Part model, mm, in its own coordinate system. A direction names the side the tool comes from. Give positions to 0.01 mm unless a question says otherwise; leave off trailing zeros. Order: outer loops, then holes, each group sorted by start corner. A loop starts at its lowest first (then second) coordinate and runs counter-clockwise, first axis right, second up. Notation, with made-up numbers: M 10,23.5 L 45,23.5 A18 ccw 45,46.5 Z; hole C -15,48 d3. An arc over 180 degrees is marked long. Answer as a JSON object with one key per item and string values.
from build123d import *

# Parameters (mm, degrees)
HEX_START   = -2.8194
HEX_2_DEPTH = 2.8194


with BuildPart() as part:
    # BodySke → BaseBody (revolve)
    with BuildSketch(Plane.XY, mode=Mode.PRIVATE) as basebody_sk:
        Polygon((0, 0), (0, 6.61924), (0.127, 6.61924), (4.089144883, 3.175), (24.64435, 3.175), (25.4, 2.41935), (25.4, 0), align=None)
    revolve(basebody_sk.sketch.rotate(Axis((0, 0, 0), (1, 0, 0)), 90), axis=Axis((0, 0, 0), (1, 0, 0)))

    # Hex 2: read off the stored shape, not the designer's step
    # Hex 2 outline → Hex 2 (cut)
    with BuildSketch(Plane.ZY.offset(HEX_START)):
        Polygon((-1.9812, -1.143846353), (0, -2.287692707), (1.9812, -1.143846353), (1.9812, 1.143846353), (0, 2.287692707), (-1.9812, 1.143846353), align=None)
    extrude(amount=HEX_2_DEPTH, mode=Mode.SUBTRACT)

    # Hex 2 2 outline → Hex 2 2 (revolve, cut)
    with BuildSketch(Plane.YX):
        Polygon((1.9812, 2.8194), (0, 3.963246353), (0, 2.8194), align=None)
    revolve(axis=Axis((0, 0, 0), (1, 0, 0)), mode=Mode.SUBTRACT)


solid = part.part
1. Probe line 1 along X through (y, z) = (-2, 0); line 2 along Y through (x, z) = (1.75, 0.5); line 3 along Y through (x, z) = (22, 1.25). List the from-to ranges inside material, lowest first.
Worked answers:
{"line 1": "x = 2.82 to 25.4", "line 2": "y = -5.18 to -2, 2 to 5.18", "line 3": "y = -2.92 to 2.92"}
2. Pin check, flat tips, straight feed: P1, Ø3, axis at x = 12.5, y = 3.5, coming from the -Z side; P2, Ø2, axis at x = 16.5, y = 0, coming from the -Z side (3 decimals); P3, Ø1, axis at x = 21, z = -1.5, coming from the -Y side. Stop position of each tip, or through.
Worked answers:
{"P1": "stops at z = -2.47", "P2": "stops at z = -3.175", "P3": "stops at y = -3.01"}
3. Two-plate mould, pull along Y, no slides. Class faces 3 (the cylindrical face through (14.51, 1.93, -2.52)), 4 (the flat face through (25.4, 0, 0)), 5 (the flat face through (1.43, 1.72, -0.98)): +Y half, -Y half, draft (parallel to the pull), parting line (faces both ways), or undercut.
Worked answers:
{"face 3": "parting line", "face 4": "draft", "face 5": "undercut"}
4. Cut at A-A on x = 2.5. Give the cut face in (y, z), plus the area to 3 significant figures.
Worked answers:
{"outline": "C 0,0 d9.11; hole M -2.29,0 L -1.14,-1.98 L 1.14,-1.98 L 2.29,0 L 1.14,1.98 L -1.14,1.98 Z", "area": "51.6 mm^2"}
5. Which spindle directions (+Z, -Z, +X, -X, +Y, -Y) get a long thin tool onto all of the face, cutting with end or side? Do faces 1 (the flat face through (0, -2, -1)), 2 (the flat face through (1.43, -1.71, -1)). Say none if no direction does.
Worked answers:
{"face 1": "+Z, -Z, -X, +Y, -Y", "face 2": "-X"}
6. Cut at B-B on x = 13. Give the cut face in (y, z) (3 decimals).
Worked answers:
{"outline": "C 0,0 d6.35"}
